from build123d import *

# Parameters (mm, degrees)
SKETCH1_R           = 1.143
BOSS_EXTRUDE1_DEPTH = 3.175


with BuildPart() as part:
    # Sketch1 → Boss-Extrude1 (new body)
    with BuildSketch(Plane.XY):
        with BuildLine():
            ThreePointArc((-6.731, -2.54), (-9.271, 0), (-6.731, 2.54))
            add(Edge.make_bspline(
                [(-6.731, 2.54), (-5.187542856, 2.54), (-2.92113625, 5.080180466), (0, 5.08)],
                knots=[0, 0, 0, 0, 1, 1, 1, 1], degree=3))
            add(Edge.make_bspline(
                [(6.731, 2.54), (5.187542856, 2.54), (2.92113625, 5.080180466), (0, 5.08)],
                knots=[0, 0, 0, 0, 1, 1, 1, 1], degree=3))
            ThreePointArc((6.731, 2.54), (9.271, 0), (6.731, -2.54))
            add(Edge.make_bspline(
                [(6.731, -2.54), (5.187542856, -2.54), (2.92113625, -5.080180466), (0, -5.08)],
                knots=[0, 0, 0, 0, 1, 1, 1, 1], degree=3))
            add(Edge.make_bspline(
                [(-6.731, -2.54), (-5.187542856, -2.54), (-2.92113625, -5.080180466), (0, -5.08)],
                knots=[0, 0, 0, 0, 1, 1, 1, 1], degree=3))
        make_face()
        with Locations((6.731, 0)):
            Circle(SKETCH1_R, mode=Mode.SUBTRACT)
        with Locations((-6.731, 0)):
            Circle(SKETCH1_R, mode=Mode.SUBTRACT)
    extrude(amount=BOSS_EXTRUDE1_DEPTH)

    # Sketch4 → Revolve1 (revolve)
    with BuildSketch(Plane(origin=(0, 0, 0), x_dir=(1, 0, 0), z_dir=(0, 1, 0))):
        with BuildLine():
            Line((0, 0), (4.212113484, 0))
            ThreePointArc((4.212113484, 0), (4.078361344, 4.681844425), (0, 6.985))
            Line((0, 6.985), (0, 0))
        make_face()
    revolve(axis=Axis((0, 0, 0), (0, 0, -1)))


solid = part.part
Geometry: final body of the model. Coordinates: model frame, mm. Coordinates: 2 decimals unless noted, no trailing zeros. Loops run counter-clockwise (first coordinate to the right, second up) from the corner with the lowest first, then second, coordinate; pieces in that order, holes last. Notation, with made-up numbers: (51, 80.25) - (62, 80.25) arc R29 ccw to (62, 111.25) - close; hole circle Ø8 at (-15, 54). An arc over 180 degrees is marked (long way). One line per question, with ' | ' between items. Start each with the question number.
(1) Draft query along Z for faces 1 (the cylindrical face through (-5.675, -0.438, 1.565)), 2 (the flat face through (4.3, 1.2, 0)), 3 (the flat face through (0, 0, 3.175)). Return one class per face: +Z half, -Z half, draft (parallel to the pull), parting line (faces both ways), or undercut.
(2) Cut plane B-B on y = 2. Output: boundary loops of the cut face in (x, z) (1 decimal), and give its area (3 significant figures).
(3) First-contact query: pin 1 (2.5 mm diameter, centred on x = 6.731, y = 0, fed in from -Z); pin 2 (4 mm diameter, centred on x = 1, z = -2.5, fed in from +Y); pin 3 (2 mm diameter, centred on x = 5.5, z = 1.5, fed in from +Y). Flat tips, straight axial feed; report the tip coordinate or a pass-through.
(4) Cut plane C-C on z = -2.75. Output: boundary loops of the cut face in (x, y).
(5) Cut plane A-A on y = 0. Output: boundary loops of the cut face in (x, z) (1 decimal).
(6) Ray query, L1, parallel to X at y = -0.75, z = 2; L2, parallel to Z at x = 7.75, y = -1.25 (3 decimals); L3, parallel to Y at x = 6, z = 2.75. Return the intervals inside material, ascending. Write a range as from..to.
(7) Cut plane D-D on y = -1.5. Output: boundary loops of the cut face in (x, z) (1 decimal).
Here are the results:
1) face 1: draft | face 2: undercut | face 3: +Z half
2) outline: (-8.3, 0) - (-3.7, 0) arc R4.3 ccw (long way) to (3.7, 0) - (8.3, 0) - (8.3, 3.2) - (-8.3, 3.2) - close | area: 100 mm²
3) pin 1: z = 0 | pin 2: y = 4.76 | pin 3: y = 3.46
4) outline: circle Ø9.47 at (0, 0)
5) outline: (-9.3, 0) - (-7.9, 0) - (-7.9, 3.2) - (-9.3, 3.2) - close; (-5.6, 0) - (-4.2, 0) arc R4.8 ccw (long way) to (4.2, 0) - (5.6, 0) - (5.6, 3.2) - (-5.6, 3.2) - close; (7.9, 0) - (9.3, 0) - (9.3, 3.2) - (7.9, 3.2) - close
6) L1: -9.16..-7.59, -5.87..5.87, 7.59..9.16 | L2: 0..3.175 | L3: -2.69..-0.88, 0.88..2.69
7) outline: (-8.8, 0) - (-3.9, 0) arc R4.5 ccw (long way) to (3.9, 0) - (8.8, 0) - (8.8, 3.2) - (-8.8, 3.2) - close
